Can you work these out from the drawing? Everything is in mm from the part's minimum corner. A direction names the side the tool comes from. Give positions to 0.01 mm unless a question says otherwise; leave off trailing zeros. Write each loop counter-clockwise with the first axis right and the second up, starting at its lowest first coordinate (ties: lowest second). Pieces come first, ordered by that corner, then holes. Notation, with made-up numbers: (70.25, 55.25) - (77.25, 55.25) arc R16 ccw to (77.25, 85.25) - close; hole circle Ø7 at (45.25, 42). An arc over 180 degrees is marked (long way). Use a Markdown table: item, result.
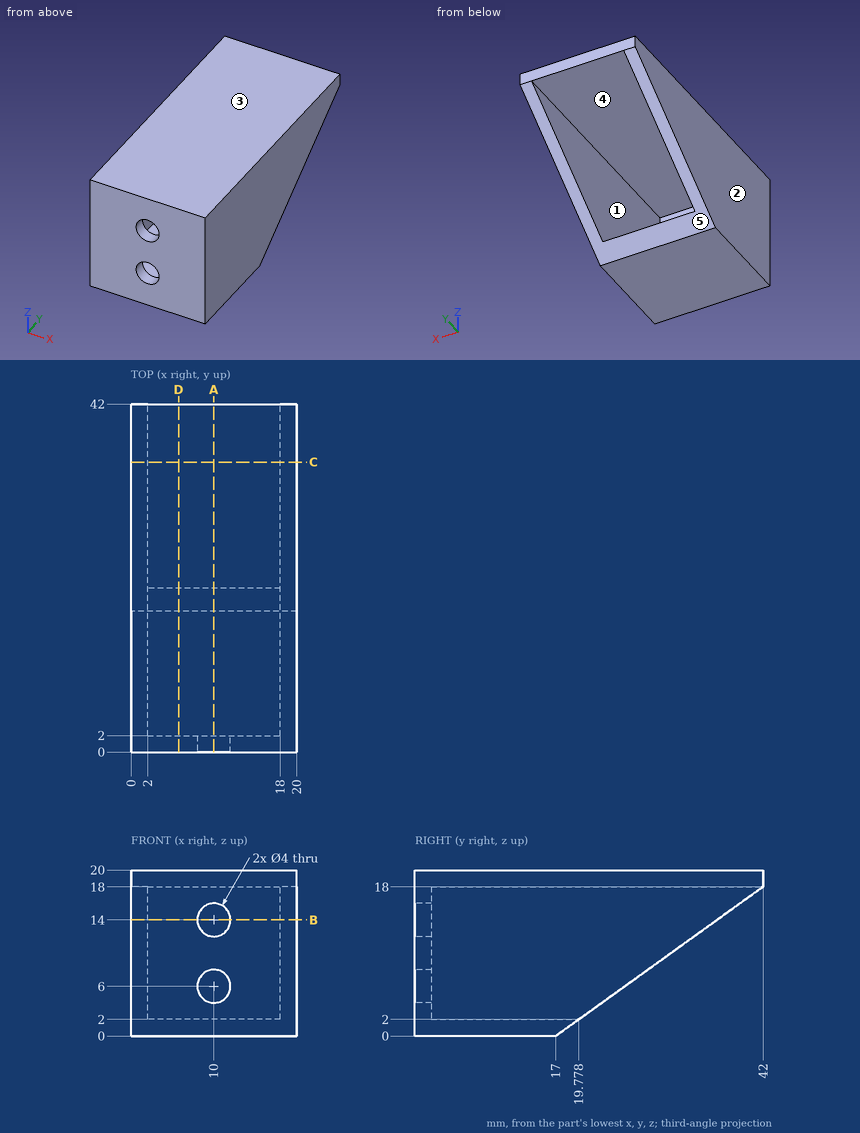
Item 1: For the marked faces 4 and 5, which set-ups out of +Z, -Z, +X, -X, +Y, -Y let a thin tool reach every point of the face, with its end or its side?
Values:
| item | result |
|---|---|
| face 4 | +Y |
| face 5 | -Z, +X, -X, +Y |
Item 2: Will these pins go through, and if not, where does the flat tip stop? pin 1 Ø1 at (x, y) = (13.5, 26) entering from -Z; pin 2 Ø5 at (x, z) = (12.5, 9) entering from +Y; pin 3 Ø12 at (x, y) = (11, 9.5) entering from -Z.
Values:
| item | result |
|---|---|
| pin 1 | stops at z = 18 |
| pin 2 | stops at y = 2 |
| pin 3 | stops at z = 0 |
Item 3: Thinking about a two-plate mould opening in Z: for the marked faces 1, 2 and 3, which applies, +Z half, -Z half, draft (parallel to the pull), parting line (faces both ways), or undercut?
Values:
| item | result |
|---|---|
| face 1 | undercut |
| face 2 | draft |
| face 3 | +Z half |
Item 4: If we section it at A-A, the plane x = 10: Write out the boundary of the cut face in (y, z), plus the area to 3 significant figures.
Values:
| item | result |
|---|---|
| outline | (0, 0) - (17, 0) - (19.78, 2) - (2, 2) - (2, 4) - (0, 4) - close; (0, 8) - (2, 8) - (2, 12) - (0, 12) - close; (0, 16) - (2, 16) - (2, 18) - (42, 18) - (42, 20) - (0, 20) - close |
| area | 137 mm2 |
Item 5: If we section it at B-B, the plane z = 14: Write out the boundary of the cut face in (x, y), plus the area to 3 significant figures.
Values:
| item | result |
|---|---|
| outline | (0, 0) - (8, 0) - (8, 2) - (2, 2) - (2, 36.44) - (0, 36.44) - close; (12, 0) - (20, 0) - (20, 36.44) - (18, 36.44) - (18, 2) - (12, 2) - close |
| area | 170 mm2 |
Item 6: I need wall thicknesses on line 1 along Z through (x, y) = (10, 1.55); line 2 along X through (y, z) = (26, 9.25); line 3 along Y through (x, z) = (15.25, 17). Which ranges of each line are inside material? Lowest first, please. Write a range as [from, to].
Values:
| item | result |
|---|---|
| line 1 | z = [0, 4], [8, 12], [16, 20] |
| line 2 | x = [0, 2], [18, 20] |
| line 3 | y = [0, 2] |
Item 7: If we section it at D-D, the plane x = 5.75: Write out the boundary of the cut face in (y, z), plus the area to 3 significant figures.
Values:
| item | result |
|---|---|
| outline | (0, 0) - (17, 0) - (19.78, 2) - (2, 2) - (2, 18) - (42, 18) - (42, 20) - (0, 20) - close |
| area | 153 mm2 |
Item 8: If we section it at C-C, the plane y = 35: Write out the boundary of the cut face in (x, z).
Values:
| item | result |
|---|---|
| outline | (0, 12.96) - (2, 12.96) - (2, 18) - (18, 18) - (18, 12.96) - (20, 12.96) - (20, 20) - (0, 20) - close |
